The figure shows three views and two pictorial views of one solid part (mm, origin at its lowest corner). Answer the questions. A direction names the side the tool comes from. Coordinates: 2 decimals unless noted, no trailing zeros. Write each loop counter-clockwise with the first axis right and the second up, starting at its lowest first coordinate (ties: lowest second). Pieces come first, ordered by that corner, then holes. Notation, with made-up numbers: M 13,8.5 L 29,8.5 A24 cw 29,37.5 Z; hole C 60,36 d1. An arc over 180 degrees is marked long. Use a Markdown table: item, result. Add a question column.
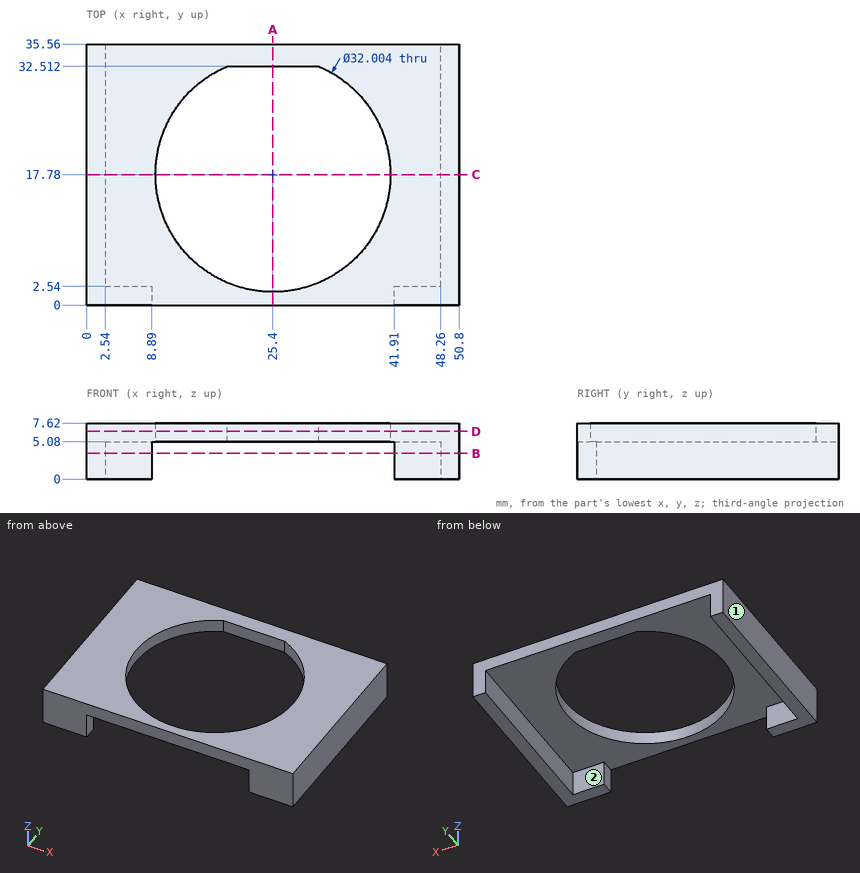
Item 1: For the marked faces 1 and 2, determine the directions among +Z, -Z, +X, -X, +Y, -Y from which every point of the face is accessible in a straight line to the end or side of a thin tool.
Item 2: Find section B-B on z = 3.5. Give the vertices of the cut face in (x, y), then the cut area to 3 significant figures.
Item 3: Consider probe 1 along X at (y, z) = (9, 3.5); probe 2 along X at (y, z) = (17.78, 6.45); probe 3 along Y at (x, z) = (25.4, 6.1). Determine where each line is inside the solid, lowest interval first.
Item 4: Find section A-A on x = 25.4. Give the vertices of the cut face in (y, z).
Item 5: Each of these flat-tipped pins is pushed along its axis until it touches: pin 1 (4 mm diameter, centred on x = 6, z = 3, fed in from +Y); pin 2 (8 mm diameter, centred on x = 44, y = 25, fed in from -Z). Where does it stop, or does it pass through?
Item 6: Find section C-C on y = 17.78. Give the vertices of the cut face in (x, z).
Item 7: Find section D-D on z = 6.5. Give the vertices of the cut face in (x, y), then the cut area to 3 significant figures.
Geometry says:
| question | item | result |
|---|---|---|
| 1 | face 1 | +Z, -Z, -X, +Y, -Y |
| 1 | face 2 | -Z, +Y |
| 2 | outline | M 0,0 L 8.89,0 L 8.89,2.54 L 2.54,2.54 L 2.54,35.56 L 0,35.56 Z; M 41.91,0 L 50.8,0 L 50.8,35.56 L 48.26,35.56 L 48.26,2.54 L 41.91,2.54 Z |
| 2 | area | 213 mm2 |
| 3 | probe 1 | x = 0 to 2.54, 48.26 to 50.8 |
| 3 | probe 2 | x = 0 to 9.4, 41.4 to 50.8 |
| 3 | probe 3 | y = 0 to 1.78, 32.51 to 35.56 |
| 4 | outline | M 0,5.08 L 1.78,5.08 L 1.78,7.62 L 0,7.62 Z; M 32.51,5.08 L 35.56,5.08 L 35.56,7.62 L 32.51,7.62 Z |
| 5 | pin 1 | stops at y = 2.54 |
| 5 | pin 2 | stops at z = 5.08 |
| 6 | outline | M 0,0 L 2.54,0 L 2.54,5.08 L 9.4,5.08 L 9.4,7.62 L 0,7.62 Z; M 41.4,5.08 L 48.26,5.08 L 48.26,0 L 50.8,0 L 50.8,7.62 L 41.4,7.62 Z |
| 7 | outline | M 0,0 L 50.8,0 L 50.8,35.56 L 0,35.56 Z; hole M 19.15,32.51 A16 ccw long 31.65,32.51 Z |
| 7 | area | 1,010 mm2 |
